from build123d import *

# Parameters (mm, degrees)
EXTRUDE_1_DEPTH     = 20
SKETCH_3_R          = 4.5
CUT_EXTRUDE_2_DEPTH = 20
CHAMFER_1_SIZE      = 5
CHAMFER_2_SIZE      = 5


with BuildPart() as part:
    # 草图1 → 凸台-拉伸1 (new body)
    with BuildSketch(Plane.XY):
        with BuildLine():
            Line((0, 5), (0, 30))
            Line((0, 30), (10, 30))
            Line((10, 30), (10, 21.3))
            ThreePointArc((10, 21.3), (14.188611699, 9.052551286), (25, 1.935083269))
            Line((25, 1.935083269), (25, 0))
            Line((25, 0), (6.25, 0))
            Line((6.25, 0), (0, 0))
            Line((0, 0), (0, -20))
            Line((0, -20), (-5, -20))
            Line((-5, -20), (-5, 5))
            Line((-5, 5), (0, 5))
        make_face()
    extrude(amount=EXTRUDE_1_DEPTH)

    # 草图3 → 切除-拉伸2 (cut)
    with BuildSketch(Plane.ZY.offset(5)):
        with Locations((10, -10)):
            Circle(SKETCH_3_R)
    extrude(amount=-CUT_EXTRUDE_2_DEPTH, mode=Mode.SUBTRACT)

    # 倒角1
    chamfer_1_edges = [part.edges().sort_by_distance(p)[0] for p in [
        (0, 5, 10),
    ]]
    chamfer(chamfer_1_edges, length=CHAMFER_1_SIZE - 0.0001)  # a hair under: the kernel refuses the full size

    # 倒角2
    chamfer_2_edges = [part.edges().sort_by_distance(p)[0] for p in [
        (0, 30, 10),
    ]]
    chamfer(chamfer_2_edges, length=CHAMFER_2_SIZE)


solid = part.part
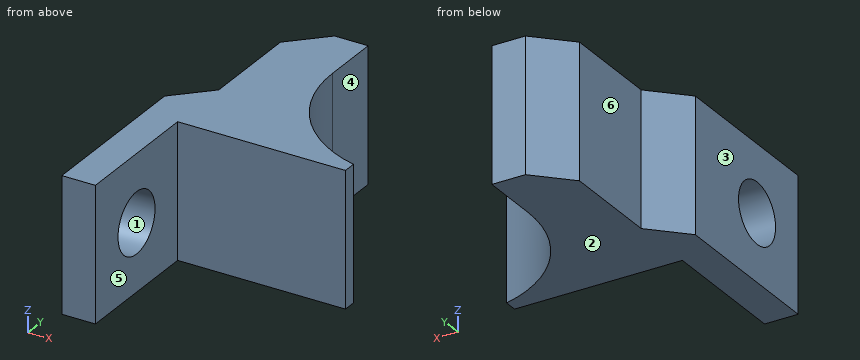
Can you work these out from the model? Positions are in its coordinate system, mm. Face numbers are marked on the shaded views. A direction names the side the tool comes from. Coordinates: 2 decimals unless noted, no trailing zeros. Write each loop counter-clockwise with the first axis right and the second up, starting at its lowest first coordinate (ties: lowest second). Pieces come first, ordered by that corner, then holes. Notation, with made-up numbers: M -27,-10.5 L -1,-10.5 A7 cw -1,2.5 Z; hole C 62,61 d11. An arc over 180 degrees is marked long. Use one line per item in the form item = value.
Q1. For the marked faces 4, 5 and 6, which set-ups out of +Z, -Z, +X, -X, +Y, -Y let a thin tool reach every point of the face, with its end or its side?
Model answer:
face_4 = +Z, -Z, +X, +Y
face_5 = +Z, -Z, +X, -Y
face_6 = +Z, -Z, -X, +Y
Q2. We'd pull the mould along Z, two halves only. Please class the marked faces 1, 2 and 3: +Z half, -Z half, draft (parallel to the pull), parting line (faces both ways), or undercut.
Model answer:
face_1 = undercut
face_2 = -Z half
face_3 = draft
Q3. For P1, Ø6, axis at x = 18, z = 6, coming from the -Y side; P2, Ø2.5, axis at y = 24.5, z = 9.5, coming from the +X side, each with a flat end and sliding along its axis, tell me the tip position at first contact or that it passes through.
Model answer:
P1 = 0
P2 = 10
Q4. If we section it at B-B (y = -10): Write out the boundary of the cut face in (x, z), then the cut area to 3 significant figures.
Model answer:
outline = M -5,0 L 0,0 L 0,5.5 L -5,5.5 Z; M -5,14.5 L 0,14.5 L 0,20 L -5,20 Z
area = 55.0 mm^2
Q5. I need wall thicknesses on line 1 along Y through (x, z) = (-3.45, 10); line 2 along Y through (x, z) = (13.5, 6); line 3 along X through (y, z) = (-4, 1). Which ranges of each line are inside material? Lowest first, please. Write a range as from..to.
Model answer:
line_1 = -20..-14.5, -5.5..6.55
line_2 = 0..10
line_3 = -5..0
Q6. If we section it at D-D (x = 6.75): Write out the boundary of the cut face in (y, z).
Model answer:
outline = M 0,0 L 30,0 L 30,20 L 0,20 Z
